```python
from build123d import *

# Parameters (mm, degrees)
BOSS_EXTRUDE5_DEPTH = 5
SKETCH6_W           = 56
SKETCH6_H           = 56
BOSS_EXTRUDE6_DEPTH = 9
SKETCH7_R           = 19
BOSS_EXTRUDE7_DEPTH = 1.3
SKETCH8_R           = 2.5
CUT_EXTRUDE1_DEPTH  = 43
SKETCH9_R           = 3.15
BOSS_EXTRUDE8_DEPTH = 19.2


with BuildPart() as part:
    # Sketch1 → Boss-Extrude5 (new body)
    with BuildSketch(Plane(origin=(0, 0, 0), x_dir=(1, 0, 0), z_dir=(0, 1, 0))):
        with BuildLine():
            Line((-18.5, 28), (18.5, 28))
            ThreePointArc((18.5, 28), (21.282485579, 21.282485579), (28, 18.5))
            Line((28, 18.5), (28, -18.5))
            ThreePointArc((28, -18.5), (21.282485579, -21.282485579), (18.5, -28))
            Line((18.5, -28), (-18.5, -28))
            ThreePointArc((-18.5, -28), (-21.282485579, -21.282485579), (-28, -18.5))
            Line((-28, -18.5), (-28, 18.5))
            ThreePointArc((-28, 18.5), (-21.282485579, 21.282485579), (-18.5, 28))
        make_face()
    extrude(amount=BOSS_EXTRUDE5_DEPTH)

    # Sketch6 → Boss-Extrude6 (add)
    with BuildSketch(Plane(origin=(0, 5, 0), x_dir=(1, 0, 0), z_dir=(0, 1, 0))):
        Rectangle(SKETCH6_W, SKETCH6_H)
    extrude(amount=BOSS_EXTRUDE6_DEPTH)

    # Sketch7 → Boss-Extrude7 (add)
    with BuildSketch(Plane(origin=(0, 14, 0), x_dir=(1, 0, 0), z_dir=(0, 1, 0))):
        with Locations(Location((0, 0, 0), (0, 0, 270))):
            Circle(SKETCH7_R)
    extrude(amount=BOSS_EXTRUDE7_DEPTH)

    # Sketch8 → Cut-Extrude1 (cut, through all)
    with BuildSketch(Plane(origin=(0, 14, 0), x_dir=(1, 0, 0), z_dir=(0, 1, 0))):
        with Locations(Location((-23.5, 23.5, 0), (0, 0, 270))):
            Circle(SKETCH8_R)
        with Locations(Location((23.5, 23.5, 0), (0, 0, 270))):
            Circle(SKETCH8_R)
        with Locations(Location((23.5, -23.5, 0), (0, 0, 270))):
            Circle(SKETCH8_R)
        with Locations(Location((-23.5, -23.5, 0), (0, 0, 270))):
            Circle(SKETCH8_R)
    extrude(amount=-CUT_EXTRUDE1_DEPTH, mode=Mode.SUBTRACT)

    # Sketch9 → Boss-Extrude8 (add)
    with BuildSketch(Plane(origin=(0, 15.3, 0), x_dir=(1, 0, 0), z_dir=(0, 1, 0))):
        with Locations(Location((0, 0, 0), (0, 0, 270))):
            Circle(SKETCH9_R)
    extrude(amount=BOSS_EXTRUDE8_DEPTH)


solid = part.part
```
The model under review builds one solid part; all positions refer to its coordinate system, in mm. A direction names the side the tool comes from. Coordinates: 2 decimals unless noted, no trailing zeros. Write each loop counter-clockwise with the first axis right and the second up, starting at its lowest first coordinate (ties: lowest second). Pieces come first, ordered by that corner, then holes.
1) The part is to be moulded in two halves that separate along X. For faces 4 (the face through (25.19, 9.56, -25.34)), 5 (the face through (-4, 15.3, 0)), 6 (the face through (21.209, 2.465, -21.357)), 7 (the face through (-21.81, 9.56, -25.34)), say which applies: pulls with the +X half, pulls with the -X half, needs draft (parallel to the pull), parting line crosses it, or undercut.
2) To check wall thickness, follow probe 1 along X at (y, z) = (8.75, 23.5); probe 2 along Z at (x, y) = (23, 12); probe 3 along Y at (x, z) = (20, -3). State the ranges of each line that lie inside material, in increasing order.
3) Clearance check with flat-ended pins moving along their axes: pin 1 Ø5 at (x, z) = (-24, 23) entering from -Y; pin 2 Ø6 at (x, z) = (-7.5, -6.5) entering from -Y; pin 3 Ø6.5 at (x, z) = (-23.5, 23.5) entering from +Y. State where each tip first meets the part, or that it passes through.
4) We need section C-C on x = 0. State the section outline as (y, z) points.
5) We need section A-A on y = 12. State the section outline as (x, z) points, then the cut area to 3 significant figures.
6) We need section B-B on z = 0. State the section outline as (x, y) points, then the cut area to 3 significant figures.
7) Machinability: for faces 1 (the face through (21.357, 2.465, 21.209)), 2 (the face through (24.2, 5, -26.5)), 3 (the face through (-7, 14, -19)), which of the approach directions +Z, -Z, +X, -X, +Y, -Y give a long, thin tool a straight path to every point of the face, cutting with its end or side? Answer none if there is none.
8) We need section D-D on x = -23.5. State the section outline as (y, z) points.
Answer list:
1. face 4: undercut
1. face 5: needs draft
1. face 6: pulls with the +X half
1. face 7: undercut
2. probe 1: x = -28 to -26, -21 to 21, 26 to 28
2. probe 2: z = -28 to -25.95, -21.05 to 21.05, 25.95 to 28
2. probe 3: y = 0 to 14
3. pin 1: stops at y = 5
3. pin 2: stops at y = 0
3. pin 3: stops at y = 14
4. outline: (0, -28) - (14, -28) - (14, -19) - (15.3, -19) - (15.3, -3.15) - (34.5, -3.15) - (34.5, 3.15) - (15.3, 3.15) - (15.3, 19) - (14, 19) - (14, 28) - (0, 28) - close
5. outline: (-28, -28) - (28, -28) - (28, 28) - (-28, 28) - close; hole circle Ø5 at (-23.5, -23.5); hole circle Ø5 at (-23.5, 23.5); hole circle Ø5 at (23.5, -23.5); hole circle Ø5 at (23.5, 23.5)
5. area: 3,060 mm2
6. outline: (-28, 0) - (28, 0) - (28, 14) - (19, 14) - (19, 15.3) - (3.15, 15.3) - (3.15, 34.5) - (-3.15, 34.5) - (-3.15, 15.3) - (-19, 15.3) - (-19, 14) - (-28, 14) - close
6. area: 954 mm2
7. face 1: +Z, +X, -Y
7. face 2: -Z, +X, -Y
7. face 3: +Y
8. outline: (0, -19.63) - (5, -19.63) - (5, -21) - (14, -21) - (14, 21) - (5, 21) - (5, 19.63) - (0, 19.63) - close; (5, -28) - (14, -28) - (14, -26) - (5, -26) - close; (5, 26) - (14, 26) - (14, 28) - (5, 28) - close
